For this review, take the finished solid that the model builds, in its own axes (mm). A direction names the side the tool comes from. Give positions to 0.01 mm unless a question says otherwise; leave off trailing zeros. Write each loop counter-clockwise with the first axis right and the second up, starting at its lowest first coordinate (ties: lowest second). Pieces come first, ordered by that corner, then holes. Notation, with made-up numbers: (67, 26.5) -> (86, 26.5) arc R25 ccw to (86, 39.5) -> close; hole circle Ø2 at (36.5, 60.5). An arc over 180 degrees is marked (long way). Return JSON: item names as keys, results as strings.
from build123d import *

# Parameters (mm, degrees)
CYLINDER007_R     = 2.2
CYLINDER007_DEPTH = 15
CYLINDER006_R     = 2.2
CYLINDER006_DEPTH = 15
CYLINDER005_R     = 4.7
CYLINDER005_DEPTH = 15
CYLINDER004_R     = 3.5
CYLINDER004_DEPTH = 15
BOX001006_W       = 40
BOX001006_H       = 20
BOX001006_DEPTH   = 10


with BuildPart() as cylinder007:
    # Cylinder007 → Cylinder007 (new body)
    with BuildSketch(Plane(origin=(33, 10, -1), x_dir=(1, 0, 0), z_dir=(0, 0, 1))):
        Circle(CYLINDER007_R)
    extrude(amount=CYLINDER007_DEPTH)


with BuildPart() as fusion004:
    # Cylinder006 → Cylinder006 (new body)
    with BuildSketch(Plane(origin=(7, 10, -1), x_dir=(1, 0, 0), z_dir=(0, 0, 1))):
        Circle(CYLINDER006_R)
    extrude(amount=CYLINDER006_DEPTH)

    # Fusion004: union Cylinder007
    add(cylinder007.part)


with BuildPart() as cylinder005:
    # Cylinder005 → Cylinder005 (new body)
    with BuildSketch(Plane(origin=(20, 10, 5), x_dir=(1, 0, 0), z_dir=(0, 0, 1))):
        Circle(CYLINDER005_R)
    extrude(amount=CYLINDER005_DEPTH)


with BuildPart() as fusion003:
    # Cylinder004 → Cylinder004 (new body)
    with BuildSketch(Plane(origin=(20, 10, -1), x_dir=(1, 0, 0), z_dir=(0, 0, 1))):
        Circle(CYLINDER004_R)
    extrude(amount=CYLINDER004_DEPTH)

    # Fusion003: union Cylinder005
    add(cylinder005.part)


with BuildPart() as cut004:
    # Box001006 → Box001006 (new body)
    with BuildSketch(Plane.XY):
        with Locations((20, 10)):
            Rectangle(BOX001006_W, BOX001006_H)
    extrude(amount=BOX001006_DEPTH)

    # Cut003: cut Fusion003
    add(fusion003.part, mode=Mode.SUBTRACT)

    # Cut004: cut Fusion004
    add(fusion004.part, mode=Mode.SUBTRACT)


with BuildPart() as cut004_1:
    # Cut004 placement: moved
    add(cut004.part.moved(Location((0, 0, 34))))


solid = cut004_1.part
1. For pin 1 (4 mm diameter, centred on x = 33, y = 10, fed in from -Z); pin 2 (3 mm diameter, centred on x = 21, y = 12, fed in from +Z), all flat-tipped, find the tip position at first contact; note any pin that passes through.
Results found:
{"pin 1": "passes through", "pin 2": "stops at z = 39"}
2. Add section D-D, the plane z = 43.5. State the section outline as (x, y) points, plus the area to 3 significant figures.
Results found:
{"outline": "(0, 0) -> (40, 0) -> (40, 20) -> (0, 20) -> close; hole circle Ø4.4 at (7, 10); hole circle Ø9.4 at (20, 10); hole circle Ø4.4 at (33, 10)", "area": "700 mm²"}
3. Add section A-A, the plane y = 10. State the section outline as (x, z) points.
Results found:
{"outline": "(0, 34) -> (4.8, 34) -> (4.8, 44) -> (0, 44) -> close; (9.2, 34) -> (16.5, 34) -> (16.5, 39) -> (15.3, 39) -> (15.3, 44) -> (9.2, 44) -> close; (23.5, 34) -> (30.8, 34) -> (30.8, 44) -> (24.7, 44) -> (24.7, 39) -> (23.5, 39) -> close; (35.2, 34) -> (40, 34) -> (40, 44) -> (35.2, 44) -> close"}
4. Add section C-C, the plane x = 7. State the section outline as (y, z) points, plus the area to 3 significant figures.
Results found:
{"outline": "(0, 34) -> (7.8, 34) -> (7.8, 44) -> (0, 44) -> close; (12.2, 34) -> (20, 34) -> (20, 44) -> (12.2, 44) -> close", "area": "156 mm²"}
5. For faces 1 (the cylindrical face through (30.802, 10.097, 38.93)), 2 (the cylindrical face through (15.305, 10.207, 41.465)), list the 3-axis set-ups (+Z, -Z, +X, -X, +Y, -Y) from which the entire face can be reached by the end or side of a thin tool; tool diameter is ignored.
Results found:
{"face 1": "+Z, -Z", "face 2": "+Z"}
6. The part is to be moulded in two halves that separate along Y. For faces 3 (the flat face through (20, 20, 39)), 4 (the flat face through (20, 0, 39)), 5 (the cylindrical face through (9.032, 9.157, 38.93)), 6 (the flat face through (15, 10, 44)), say which applies: +Y half, -Y half, draft (parallel to the pull), parting line (faces both ways), or undercut.
Results found:
{"face 3": "+Y half", "face 4": "-Y half", "face 5": "undercut", "face 6": "draft"}
7. To check wall thickness, follow probe 1 along X at (y, z) = (10, 40.2); probe 2 along Y at (x, z) = (20, 41.75); probe 3 along Y at (x, z) = (20, 36.6). State the ranges of each line that lie inside material, in increasing order.
Results found:
{"probe 1": "x = 0 to 4.8, 9.2 to 15.3, 24.7 to 30.8, 35.2 to 40", "probe 2": "y = 0 to 5.3, 14.7 to 20", "probe 3": "y = 0 to 6.5, 13.5 to 20"}
8. Add section B-B, the plane z = 38.25. State the section outline as (x, y) points, plus the area to 3 significant figures.
Results found:
{"outline": "(0, 0) -> (40, 0) -> (40, 20) -> (0, 20) -> close; hole circle Ø4.4 at (7, 10); hole circle Ø7 at (20, 10); hole circle Ø4.4 at (33, 10)", "area": "731 mm²"}
